Verification items for the finished model (mm, model axes). A direction names the side the tool comes from. Give positions to 0.01 mm unless a question says otherwise; leave off trailing zeros. Order: outer loops, then holes, each group sorted by start corner. A loop starts at its lowest first (then second) coordinate and runs counter-clockwise, first axis right, second up. Notation, with made-up numbers: M 26.5,42.25 L 64.5,42.25 A29 ccw 64.5,72.25 Z; hole C 40.5,88 d7. An arc over 180 degrees is marked long. Answer as a JSON object with one key per item and string values.
```python
from build123d import *

# Parameters (mm, degrees)
F0_R     = 1.6
F1_DEPTH = 3.175


with BuildPart() as f1:
    # F0 (on Top) → F1 (new body)
    with BuildSketch(Plane.XY):
        with BuildLine():
            ThreePointArc((5.5901699437, 5), (0, 7.5), (-5.5901699437, 5))
            Line((-5.5901699437, 5), (-32.6, 5))
            ThreePointArc((-32.6, 5), (-36.1355339059, 3.5355339059), (-37.6, 0))
            ThreePointArc((-37.6, 0), (-36.1355339059, -3.5355339059), (-32.6, -5))
            Line((-32.6, -5), (-5.5901699437, -5))
            ThreePointArc((-5.5901699437, -5), (0, -7.5), (5.5901699437, -5))
            Line((5.5901699437, -5), (32.6, -5))
            ThreePointArc((32.6, -5), (36.1355339059, -3.5355339059), (37.6, 0))
            ThreePointArc((37.6, 0), (36.1355339059, 3.5355339059), (32.6, 5))
            Line((32.6, 5), (5.5901699437, 5))
        make_face()
        with Locations((-33, 0)):
            Circle(F0_R, mode=Mode.SUBTRACT)
        with Locations((-23, 0)):
            Circle(F0_R, mode=Mode.SUBTRACT)
        with Locations((-13, 0)):
            Circle(F0_R, mode=Mode.SUBTRACT)
        Polygon((-2.3131272616, 1.150841372), (-2.4811892868, 1.651717782), (-1.9542535042, 1.6899369317), (-1.992472654, 2.2168727143), (-1.4725868119, 2.1228475389), (-1.3785616365, 2.6427333809), (-0.8983920744, 2.4223718279), (-0.6780305213, 2.90254139), (-0.2677480588, 2.5696895861), (0.0651037451, 2.9799720486), (0.379719552, 2.555544297), (0.8041473037, 2.8701601039), (1.0033279869, 2.380824761), (1.4926633298, 2.5800054442), (1.5638936344, 2.0565092492), (2.0873898293, 2.1277395538), (2.0261940932, 1.6029756981), (2.5509579489, 1.5417799619), (2.3611813253, 1.0487212884), (2.8542399989, 0.8589446648), (2.547806851, 0.4285718633), (2.9781796525, 0.1221387154), (2.574344302, -0.2185063082), (2.9149893256, -0.6223416587), (2.4391262327, -0.8518549247), (2.6686394987, -1.3277180175), (2.1506488918, -1.4316783634), (2.2546092377, -1.9496689703), (1.7270383715, -1.9215441851), (1.6989135863, -2.4491150513), (1.1949116786, -2.2906723188), (1.0364689461, -2.7946742265), (0.5877042905, -2.5158690862), (0.3088991502, -2.9646337418), (-0.0564307197, -2.5829845462), (-0.4380799154, -2.9483144161), (-0.6970199802, -2.4878015876), (-1.1575328087, -2.7467416524), (-1.2938129119, -2.2363009057), (-1.8042536586, -2.3725810089), (-1.80931082, -1.8442852134), (-2.3376066155, -1.8493423749), (-2.2111230752, -1.3363862984), (-2.7240791517, -1.209902758), (-2.4740023355, -0.7445173173), (-2.9393877762, -0.4944405012), (-2.5814309304, -0.105867575), (-2.9700038565, 0.2520892708), (-2.5266587261, 0.5394342163), (-2.8140036716, 0.9827793468), align=None, mode=Mode.SUBTRACT)
        with Locations((13, 0)):
            Circle(F0_R, mode=Mode.SUBTRACT)
        with Locations((23, 0)):
            Circle(F0_R, mode=Mode.SUBTRACT)
        with Locations((33, 0)):
            Circle(F0_R, mode=Mode.SUBTRACT)
    extrude(amount=F1_DEPTH)


solid = f1.part
```
Q1. Section check A-A on x = 13. Record the cut outline in (y, z) (3 decimals), then the cut area to 3 significant figures.
Resolved:
{"outline": "M -5,0 L -1.6,0 L -1.6,3.175 L -5,3.175 Z; M 1.6,0 L 5,0 L 5,3.175 L 1.6,3.175 Z", "area": "21.6 mm²"}
Q2. Section check C-C on x = -18. Record the cut outline in (y, z) (3 decimals), then the cut area to 4 significant figures.
Resolved:
{"outline": "M -5,0 L 5,0 L 5,3.175 L -5,3.175 Z", "area": "31.75 mm²"}
Q3. Tool access check on faces 5 (the face through (-19, -5, 2)), 6 (the face through (-14.6, 0.07, 1.57)), 7 (the face through (19, 5, 2)), 8 (the face through (19, -5, 2)), 9 (the face through (-19, 5, 2)). Record the directions out of +Z, -Z, +X, -X, +Y, -Y that give a thin tool (end or side, any length) a straight path to the whole face; none if there is none.
Resolved:
{"face 5": "+Z, -Z, -X, -Y", "face 6": "+Z, -Z", "face 7": "+Z, -Z, +X, +Y", "face 8": "+Z, -Z, +X, -Y", "face 9": "+Z, -Z, -X, +Y"}
Q4. Release check for a two-part mould opening along X. For faces 1 (the face through (0.1, 7.5, 1.6)), 2 (the face through (-34.6, 0.07, 1.57)), 3 (the face through (31.4, 0.07, 1.57)), 4 (the face through (-1, -3, 0)) record: +X half, -X half, draft (parallel to the pull), parting line (faces both ways), or undercut.
Resolved:
{"face 1": "parting line", "face 2": "undercut", "face 3": "undercut", "face 4": "draft"}
Q5. Section check D-D on y = 6.75. Record the cut outline in (x, z) (3 decimals), then the cut area to 3 significant figures.
Resolved:
{"outline": "M -3.269,0 L 3.269,0 L 3.269,3.175 L -3.269,3.175 Z", "area": "20.8 mm²"}
Q6. Material ranges on L1, parallel to Y at x = -23, z = 2.4; L2, parallel to X at y = 2.75, z = 2.3; L3, parallel to Y at x = 6, z = 1.9, recorded low to high.
Resolved:
{"L1": "y = -5 to -1.6, 1.6 to 5", "L2": "x = -36.78 to -0.75, -0.49 to -0.12, 0.24 to 0.64, 0.85 to 36.78", "L3": "y = -5 to 5"}
Q7. Gauge pin test, flat ends, axial feed: pin 1 Ø2.5 at (x, y) = (-23, 0) entering from +Z; pin 2 Ø1 at (y, z) = (3, 1.5) entering from -X; pin 3 Ø1 at (x, z) = (-17, 2) entering from +Y; pin 4 Ø1.6 at (x, z) = (-25.5, 1) entering from -Y. Record the tip position at first contact, or that the pin passes through.
Resolved:
{"pin 1": "passes through", "pin 2": "stops at x = -36.93", "pin 3": "stops at y = 5", "pin 4": "stops at y = -5"}
Q8. Section check B-B on z = 1.55. Count the separate pieces of the cut face and the enclosed holes in it, then the cut area to 3 significant figures.
Resolved:
{"separate pieces": "1", "enclosed holes": "7", "area": "697 mm²"}
